Here's the drawing with two shaded views (mm, measured from the low corner). I have some questions. A direction names the side the tool comes from. Give positions to 0.01 mm unless a question says otherwise; leave off trailing zeros. Write each loop counter-clockwise with the first axis right and the second up, starting at its lowest first coordinate (ties: lowest second). Pieces come first, ordered by that corner, then holes. Notation, with made-up numbers: M 62.25,39 L 114.25,39 A16 ccw 114.25,47 Z; hole C -20,37 d4. An arc over 180 degrees is marked long. Answer as a JSON object with one key per item and string values. Group by question number.
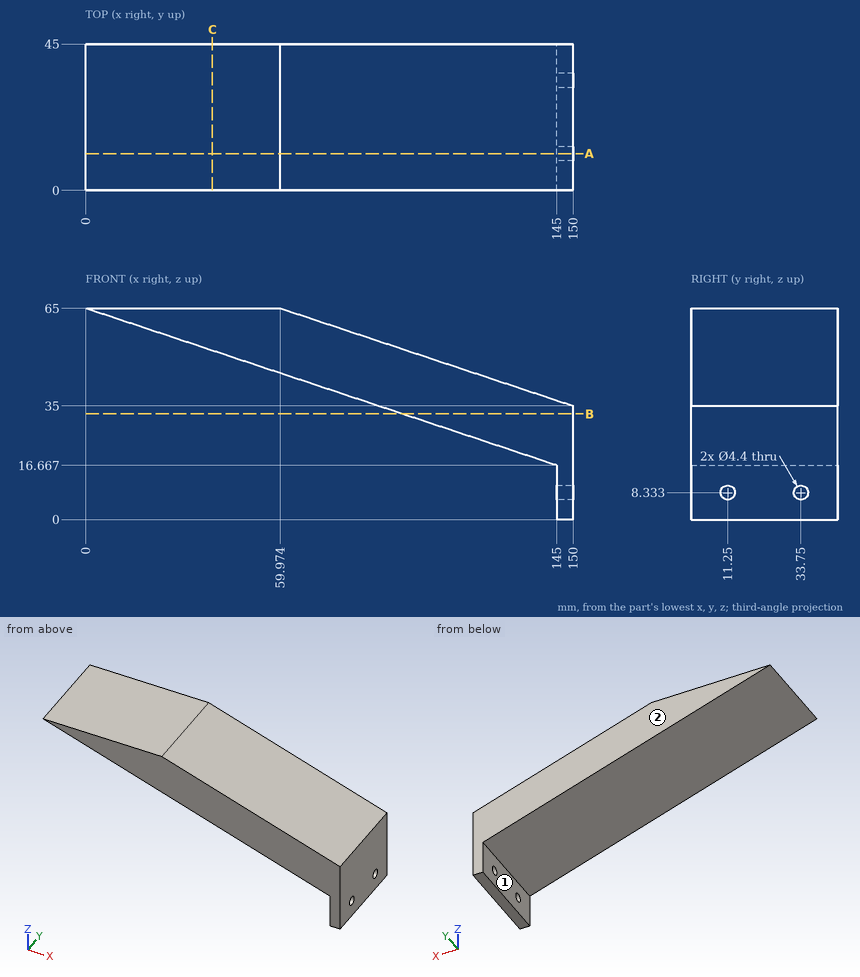
1) Please list where these lines run through material, in increasing order: line 1 along X through (y, z) = (26, 10); line 2 along Z through (x, y) = (119, 10.5); line 3 along Z through (x, y) = (147, 33) (1 decimal). Write a range as from..to.
2) If we section it at C-C, the plane x = 39: List the corners of the cut face in (y, z) for me.
3) For the marked faces 1 and 2, which set-ups out of +Z, -Z, +X, -X, +Y, -Y let a thin tool reach every point of the face, with its end or its side?
4) If we section it at A-A, the plane y = 11.25: List the corners of the cut face in (x, z) for me.
5) If we section it at B-B, the plane z = 32.5: List the corners of the cut face in (x, y) for me.
6) I'm going to push flat-ended pins straight in: pin 1 (4 mm diameter, centred on x = 131.5, y = 30.5, fed in from +Z); pin 2 (2 mm diameter, centred on x = 93.5, y = 21.5, fed in from -Z); pin 3 (3 mm diameter, centred on x = 68, y = 20, fed in from -Z). Where does each tip first touch, or does it pass through?
Taken from the geometry:
{
 "1": {"line 1": "145..150", "line 2": "25.33..45.33", "line 3": "0..6.3, 10.4..36"},
 "2": {"outline": "M 0,52 L 45,52 L 45,65 L 0,65 Z"},
 "3": {"face 1": "-Z, -X, +Y, -Y", "face 2": "+Z, -Z, +X, -X, +Y"},
 "4": {"outline": "M 0,65 L 145,16.67 L 145,10.53 L 150,10.53 L 150,35 L 59.97,65 Z; M 145,0 L 150,0 L 150,6.13 L 145,6.13 Z"},
 "5": {"outline": "M 97.5,0 L 150,0 L 150,45 L 97.5,45 Z"},
 "6": {"pin 1": "z = 41.83", "pin 2": "z = 33.5", "pin 3": "z = 41.83"}
}
